```python
from build123d import *

# Parameters (mm, degrees)
SKETCH_1_W               = 80
SKETCH_1_H               = 80
EXTRUDE_1_DEPTH          = 145
FILLET_1_R               = 10
SKETCH_2_R               = 7
EXTRUDE_2_DEPTH          = 40
SKETCH_3_R               = 3.271360977
CUT_EXTRUDE_1_DEPTH      = 10
PATTERN_CIRCULAR_1_COUNT = 3


with BuildPart() as part:
    # Эскиз1 → Бобышка-Вытянуть1 (new body)
    with BuildSketch(Plane.XY):
        with Locations((-16.484717947, -21.221052632)):
            Rectangle(SKETCH_1_W, SKETCH_1_H)
    extrude(amount=EXTRUDE_1_DEPTH)

    # Скругление1
    fillet_1_edges = [part.edges().sort_by_distance(p)[0] for p in [
        (-56.484717947, 18.778947368, 72.5),
        (23.515282053, 18.778947368, 72.5),
        (23.515282053, -61.221052632, 72.5),
        (-56.484717947, -61.221052632, 72.5),
    ]]
    fillet(fillet_1_edges, radius=FILLET_1_R)

    # Эскиз2 → Бобышка-Вытянуть2 (add)
    with BuildSketch(Plane(origin=(0, 0, 0), x_dir=(-1, 0, 0), z_dir=(0, 0, -1))):
        with Locations((16.484717947, -21.221052632)):
            Circle(SKETCH_2_R)
    extrude(amount=EXTRUDE_2_DEPTH)

    # Эскиз3 → Вырез-Вытянуть1 (cut)
    with BuildSketch(Plane(origin=(0, 0, 0), x_dir=(-1, 0, 0), z_dir=(0, 0, -1))):
        with Locations((17.021835437, 8.778947368)):
            Circle(SKETCH_3_R)
    cut_extrude_1 = extrude(amount=-CUT_EXTRUDE_1_DEPTH, mode=Mode.SUBTRACT)

    # Круговой массив1: Вырез-Вытянуть1 ×3 about axis
    pattern_circular_1_axis = Axis((-16.484717947, -21.221052632, 0), (0, 0, 1))
    for i in range(1, PATTERN_CIRCULAR_1_COUNT):
        add(cut_extrude_1.rotate(pattern_circular_1_axis, i * 360 / PATTERN_CIRCULAR_1_COUNT), mode=Mode.SUBTRACT)


solid = part.part
```
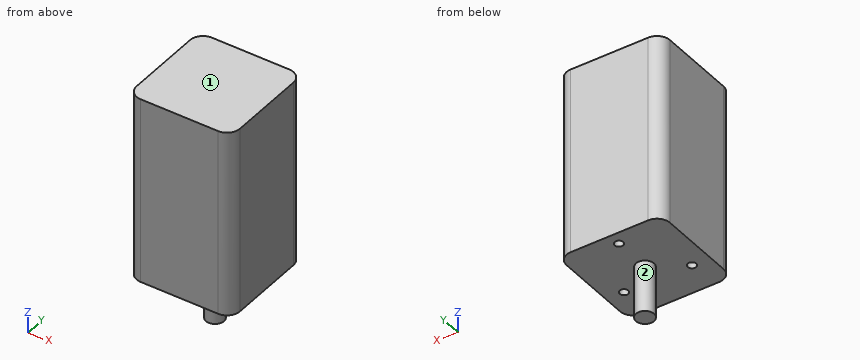
For this review, take the finished solid that the model builds, in its own axes (mm). Face numbers are marked on the shaded views. A direction names the side the tool comes from. Round coordinates to 2 decimals unless told otherwise and drop trailing zeros. Write each loop counter-clockwise with the first axis right and the second up, starting at its lowest first coordinate (ties: lowest second). Pieces come first, ordered by that corner, then holes. Notation, with made-up numbers: (39, 56) -> (44, 56) arc R12 ccw to (44, 61) -> close; hole circle Ø11 at (88.25, 68). An arc over 180 degrees is marked (long way). One line per question, with ' | ' between items. Start each with the question number.
(1) Insertion check: P1, Ø10.5, axis at x = -17.02, y = 8.78, coming from the -Z side; P2, Ø2, axis at x = -17.5, z = -19.5, coming from the +Y side; P3, Ø3.5, axis at x = -16.5, y = 8.5, coming from the -Z side. Each pin has a flat end and moves straight along its axis. Give the tip position at first contact, or say it passes through.
(2) For line 1 along Z through (x, y) = (4, -28); line 2 along Y through (x, z) = (-40, 7); line 3 along X through (y, z) = (14, 31), list the stretches that pass through material, from the lowest coordinate up. Write a range as from..to.
(3) Add section B-B, the plane x = -11.5. Write out the cut boundary in (y, z), plus the area to 3 significant figures.
(4) Add section D-D, the plane y = -9.5. Write out the cut boundary in (x, z), plus the area to 3 significant figures.
(5) Add section A-A, the plane y = -36.5. Write out the cut boundary in (x, z).
(6) Tool access review of the marked faces 1 and 2: name each direction out of +Z, -Z, +X, -X, +Y, -Y from which nothing blocks a thin tool from reaching the whole face with its end or side.
(7) Add section C-C, the plane x = 9.5. Write out the cut boundary in (y, z), plus the area to 3 significant figures.
Answer list:
1) P1: z = 0 | P2: y = -14.22 | P3: z = 10
2) line 1: 0..145 | line 2: -61.22..-39.11, -34.26..18.78 | line 3: -55.01..22.04
3) outline: (-61.22, 0) -> (-26.14, 0) -> (-26.14, -40) -> (-16.31, -40) -> (-16.31, 0) -> (18.78, 0) -> (18.78, 145) -> (-61.22, 145) -> close | area: 12,000 mm²
4) outline: (-56.48, 0) -> (23.52, 0) -> (23.52, 145) -> (-56.48, 145) -> close | area: 11,600 mm²
5) outline: (-56.48, 0) -> (-45.46, 0) -> (-45.46, 10) -> (-38.93, 10) -> (-38.93, 0) -> (6.58, 0) -> (6.58, 10) -> (12.95, 10) -> (12.95, 0) -> (23.52, 0) -> (23.52, 145) -> (-56.48, 145) -> close
6) face 1: +Z, +X, -X, +Y, -Y | face 2: -Z
7) outline: (-61.22, 0) -> (-39.02, 0) -> (-39.02, 10) -> (-32.5, 10) -> (-32.5, 0) -> (18.78, 0) -> (18.78, 145) -> (-61.22, 145) -> close | area: 11,500 mm²
